The listing builds one solid part. Answer for the finished solid, in the listing's coordinates (mm). Coordinates: 2 decimals unless noted, no trailing zeros. Order: outer loops, then holes, each group sorted by start corner. A loop starts at its lowest first (then second) coordinate and runs counter-clockwise, first axis right, second up.
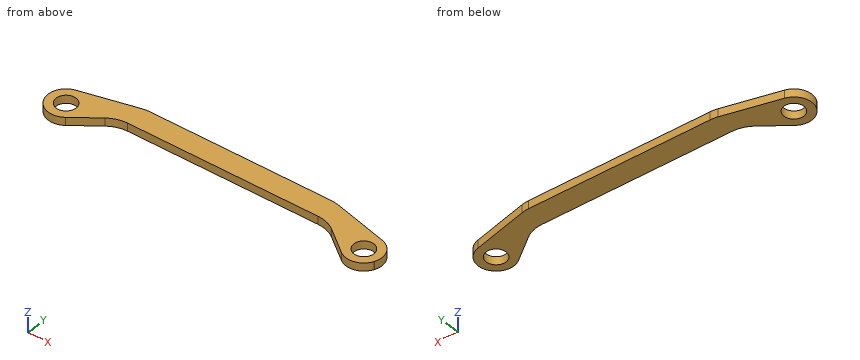
from build123d import *

# Parameters (mm, degrees)
SKETCH_1_R          = 4.4
EXTRUDE_1_DEPTH     = 4
SKETCH_2_R          = 5
CUT_EXTRUDE_1_DEPTH = 158.863865621


with BuildPart() as part:
    # 草图1 → 凸台-拉伸1 (new body)
    with BuildSketch(Plane.XY):
        with BuildLine():
            Line((28.880385739, 16.000002151), (119.119616625, 16.000002151))
            ThreePointArc((119.119616625, 16.000002151), (120.9433115, 15.888727315), (122.739948861, 15.556553752))
            Line((122.739948861, 15.556553752), (150.172338317, 8.733896395))
            ThreePointArc((150.172338317, 8.733896395), (156.114779707, 3.892345091), (156.171177789, -3.772512896))
            Line((156.171177789, -3.772512896), (156.085333125, -3.953149157))
            ThreePointArc((156.085333125, -3.953149157), (150.10671868, -8.749956366), (142.6, -7.2))
            Line((142.6, -7.2), (130.332298736, 2.00024794))
            ThreePointArc((130.332298736, 2.00024794), (126.075849791, 4.230314828), (121.332629297, 5.000000026))
            Line((121.332629297, 5.000000026), (26.667370753, 5.000000026))
            ThreePointArc((26.667370753, 5.000000026), (21.92415066, 4.230315582), (17.667701778, 2.000249685))
            Line((17.667701778, 2.000249685), (5.400000428, -7.199998281))
            ThreePointArc((5.400000428, -7.199998281), (-2.106718252, -8.749954647), (-8.085332697, -3.953147439))
            Line((-8.085332697, -3.953147439), (-8.171177361, -3.772511177))
            ThreePointArc((-8.171177361, -3.772511177), (-8.114780484, 3.892344299), (-2.172343294, 8.73389677))
            Line((-2.172343294, 8.73389677), (25.260054408, 15.556553977))
            ThreePointArc((25.260054408, 15.556553977), (27.056691327, 15.888727372), (28.880385739, 16.000002151))
        make_face()
        with Locations((4.28e-07, 1.719e-06)):
            Circle(SKETCH_1_R, mode=Mode.SUBTRACT)
        with Locations((148, 0)):
            Circle(SKETCH_1_R, mode=Mode.SUBTRACT)
    extrude(amount=EXTRUDE_1_DEPTH)

    # 草图2 → 切除-拉伸1 (cut, through all)
    with BuildSketch(Plane.XY.offset(4)):
        Circle(SKETCH_2_R)
        with Locations((148, 0)):
            Circle(SKETCH_2_R)
    extrude(amount=-CUT_EXTRUDE_1_DEPTH, mode=Mode.SUBTRACT)


solid = part.part
1) Section A-A (z = 2.1) is taken. Give the vertices of the cut face in (x, y), then the cut area to 3 significant figures.
2) Each of these flat-tipped pins is pushed along its axis until it touches: P1, Ø1, axis at x = 99, z = 0.5, coming from the -Y side; P2, Ø13, axis at x = 148, y = 0, coming from the -Z side; P3, Ø1, axis at y = 7.5, z = 3.5, coming from the +X side; P4, Ø5, axis at x = 49.5, y = 0.5, coming from the +Z side. Where does it stop, or does it pass through?
3) Section B-B (y = 0) is taken. Give the vertices of the cut face in (x, z), then the cut area to 3 significant figures.
4) Consider L1, parallel to X at y = -0.25, z = 3.5; L2, parallel to X at y = -3, z = 3.55; L3, parallel to Y at x = 70, z = 3.8. Determine where each line is inside the solid, lowest interval first.
5) Section D-D (x = 105) is taken. Give the vertices of the cut face in (y, z).
6) Section C-C (x = 148) is taken. Give the vertices of the cut face in (y, z).
Filled sheet:
1. outline: (-8.17, -3.77) - (-8.09, -3.95) arc R9 ccw to (5.4, -7.2) - (17.67, 2) arc R15 cw to (26.67, 5) - (121.33, 5) arc R15 cw to (130.33, 2) - (142.6, -7.2) arc R9 ccw to (156.09, -3.95) - (156.17, -3.77) arc R9 ccw to (150.17, 8.73) - (122.74, 15.56) arc R15 ccw to (119.12, 16) - (28.88, 16) arc R15 ccw to (25.26, 15.56) - (-2.17, 8.73) arc R9 ccw to start; hole circle Ø10 at (0, 0); hole circle Ø10 at (148, 0)
1. area: 1,890 mm2
2. P1: stops at y = 5
2. P2: stops at z = 0
2. P3: stops at x = 153.66
2. P4: passes through
3. outline: (-9, 0) - (-5, 0) - (-5, 4) - (-9, 4) - close; (5, 0) - (15, 0) - (15, 4) - (5, 4) - close; (133, 0) - (143, 0) - (143, 4) - (133, 4) - close; (153, 0) - (157, 0) - (157, 4) - (153, 4) - close
3. area: 112 mm2
4. L1: x = -9 to -4.99, 4.99 to 14.67, 133.33 to 143.01, 152.99 to 157
4. L2: x = -8.49 to -4, 4 to 11, 137 to 144, 152 to 156.49
4. L3: y = 5 to 16
5. outline: (5, 0) - (16, 0) - (16, 4) - (5, 4) - close
6. outline: (-9, 0) - (-5, 0) - (-5, 4) - (-9, 4) - close; (5, 0) - (9.27, 0) - (9.27, 4) - (5, 4) - close
